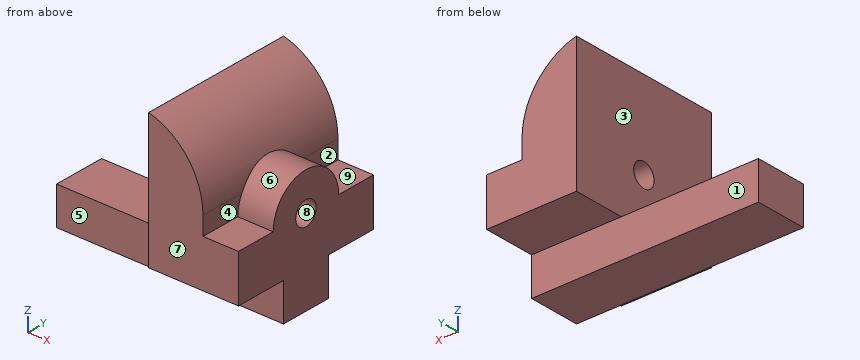
```python
from build123d import *

# Parameters (mm, degrees)
SKETCH1_R               = 5
BOSS_EXTRUDE1_DEPTH     = 15
SKETCH1_3_W             = 22
SKETCH1_3_H             = 16
BOSS_EXTRUDE2_DEPTH     = 96
SKETCH2_W               = 23
SKETCH2_H               = 57
BOSS_EXTRUDE3_DEPTH     = 66
FILLET1_R               = 30
CUT_EXTRUDE1_DEPTH      = 109.046286442
CUT_EXTRUDE1_DEPTH_BACK = 109.046286442
SKETCH1_4_R             = 5


with BuildPart() as part:
    # Sketch1 → Boss-Extrude1 (new body)
    with BuildSketch(Plane.YZ):
        with BuildLine():
            Line((16, 0), (33, 0))
            Line((33, 0), (33, -20))
            Line((33, -20), (11, -20))
            Line((11, -20), (-11, -20))
            Line((-11, -20), (-33, -20))
            Line((-33, -20), (-33, 0))
            Line((-33, 0), (-16, 0))
            ThreePointArc((-16, 0), (0, 16), (16, 0))
        make_face()
        with Locations(Location((0, 0, 0), (0, 0, 270))):
            Circle(SKETCH1_R, mode=Mode.SUBTRACT)
    extrude(amount=-BOSS_EXTRUDE1_DEPTH)

    # Sketch1<3> → Boss-Extrude2 (add)
    with BuildSketch(Plane.YZ):
        with Locations((0, -28)):
            Rectangle(SKETCH1_3_W, SKETCH1_3_H)
    extrude(amount=-BOSS_EXTRUDE2_DEPTH)

    # Sketch2 → Boss-Extrude3 (add)
    with BuildSketch(Plane(origin=(0, 33, 0), x_dir=(-1, 0, 0), z_dir=(0, 1, 0))):
        with Locations((26.5, 8.5)):
            Rectangle(SKETCH2_W, SKETCH2_H)
    extrude(amount=-BOSS_EXTRUDE3_DEPTH)

    # Fillet1
    # the kernel refuses this fillet: 30 mm, written as the material it takes off along each edge
    with BuildSketch(Plane(origin=(-15, 105.929760729, 37), x_dir=(0, 0, -1), z_dir=(0, -1, 0))) as fillet1_piece_1_section:
        with BuildLine():
            CenterArc((29.171904292, -30), FILLET1_R, 90, 76.506601178)
            Line((0, -23), (0, 0))
            Line((0, 0), (29.171904292, 0))
        make_face()
    fillet1_piece_1 = extrude(amount=211.859521458, mode=Mode.PRIVATE)
    fillet1_piece_1 = fillet1_piece_1 - Plane(origin=(-15, 0, 0), x_dir=(0, -1, 0), z_dir=(1, 0, 0)) * Cylinder(16, 541, mode=Mode.PRIVATE)
    add(fillet1_piece_1, mode=Mode.SUBTRACT)

    # Sketch1<4> → Cut-Extrude1 (cut, two sides: drawn at the far end of the back side and taken through both)
    with BuildSketch(Plane.YZ.offset(-CUT_EXTRUDE1_DEPTH_BACK)):
        with Locations(Location((0, 0, 0), (0, 0, 270))):
            Circle(SKETCH1_4_R)
    extrude(amount=CUT_EXTRUDE1_DEPTH + CUT_EXTRUDE1_DEPTH_BACK, mode=Mode.SUBTRACT)


solid = part.part
```
The model under review builds one solid part; all positions refer to its coordinate system, in mm. Face numbers are marked on the shaded views. A direction names the side the tool comes from. Coordinates: 2 decimals unless noted, no trailing zeros. Loops run counter-clockwise (first coordinate to the right, second up) from the corner with the lowest first, then second, coordinate; pieces in that order, holes last. Notation, with made-up numbers: (20.25, 2.5) -> (28.25, 2.5) arc R22 ccw to (28.25, 16.5) -> close; hole circle Ø11 at (-26, -3.5). An arc over 180 degrees is marked (long way). Answer as CSV lines item,"result".
Item 1: Machinability: for the marked faces 1, 2, 3, 4 and 5, which of the approach directions +Z, -Z, +X, -X, +Y, -Y give a long, thin tool a straight path to every point of the face, cutting with its end or side? Answer none if there is none.
Results below:
face 1,"-Z, +X, -X, +Y"
face 2,"+Z, +X, +Y"
face 3,"+Z, -X, +Y, -Y"
face 4,"+Z, +X, -Y"
face 5,"-Z, +X, -X, -Y"
Item 2: Draft analysis for pull direction Y (two halves, no side actions). For the marked faces 6, 7, 8 and 9, state which applies: +Y half, -Y half, draft (parallel to the pull), parting line (faces both ways), or undercut.
Results below:
face 6,"parting line"
face 7,"-Y half"
face 8,"undercut"
face 9,"draft"
Item 3: Take a section at B-B, the plane y = 0. State the section outline as (x, z) points, and give its area (3 significant figures).
Results below:
outline,"(-96, -36) -> (0, -36) -> (0, -5) -> (-38, -5) -> (-38, -20) -> (-96, -20) -> close; (-38, 5) -> (0, 5) -> (0, 16) -> (-16.13, 16) arc R30 ccw to (-38, 37) -> close"
area,"2,840 mm2"
Item 4: Take a section at D-D, the plane x = -80.5. State the section outline as (y, z) points.
Results below:
outline,"(-11, -36) -> (11, -36) -> (11, -20) -> (-11, -20) -> close"
Item 5: Take a section at C-C, the plane x = -28. State the section outline as (y, z) points, and give its area (3 significant figures).
Results below:
outline,"(-33, -20) -> (-11, -20) -> (-11, -36) -> (11, -36) -> (11, -20) -> (33, -20) -> (33, 32.55) -> (-33, 32.55) -> close; hole circle Ø10 at (0, 0)"
area,"3,740 mm2"
Item 6: Take a section at A-A, the plane z = -3. State the section outline as (x, y) points, and give its area (3 significant figures).
Results below:
outline,"(-38, -33) -> (0, -33) -> (0, -4) -> (-38, -4) -> close; (-38, 4) -> (0, 4) -> (0, 33) -> (-38, 33) -> close"
area,"2,200 mm2"
Item 7: For L1, parallel to Z at x = -9.5, y = 0; L2, parallel to X at y = 0.5, z = -11; L3, parallel to Y at x = -54, z = -28.5, list the stretches that pass through material, from the lowest coordinate up.
Results below:
L1,"z = -36 to -5, 5 to 16"
L2,"x = -38 to 0"
L3,"y = -11 to 11"
Item 8: Insertion check: pin 1 (16 mm diameter, centred on y = 0, z = 0, fed in from -X); pin 2 (11 mm diameter, centred on x = -12, y = 22, fed in from -Z); pin 3 (4 mm diameter, centred on x = -30, y = 9, fed in from +Z); pin 4 (13 mm diameter, centred on x = -36, z = -26, fed in from -Y). Each pin has a flat end and moves straight along its axis. Give the tip position at first contact, or say it passes through.
Results below:
pin 1,"stops at x = -38"
pin 2,"stops at z = -20"
pin 3,"stops at z = 34.87"
pin 4,"stops at y = -33"
